from build123d import *

# Parameters (mm, degrees)
BOSS_EXTRUDE1_DEPTH = 15
SCALE1_SCALE        = 0.147347741
CUT_EXTRUDE1_REACH  = 182.668
SKETCH4_R           = 2.5


with BuildPart() as part:
    # Sketch3 → Boss-Extrude1 (new body)
    with BuildSketch(Plane(origin=(0, 0, 0), x_dir=(0, 0, -1), z_dir=(1, 0, 0))):
        with BuildLine():
            Line((0, -60), (0, -86.184781703))
            ThreePointArc((0, -86.184781703), (14.644660941, -121.540120762), (50, -136.184781703))
            Line((50, -136.184781703), (73.642909299, -136.184781703))
            ThreePointArc((73.642909299, -136.184781703), (108.573727492, -150.409958986), (123.628662427, -184.991264087))
            Line((123.628662427, -184.991264087), (125.683202704, -271.037537481))
            ThreePointArc((125.683202704, -271.037537481), (116.280768167, -291.592024429), (95.295179386, -299.98831959))
            Line((95.295179386, -299.98831959), (73.775693132, -299.98831959))
            ThreePointArc((73.775693132, -299.98831959), (63.169091414, -304.381717872), (58.775693132, -314.98831959))
            Line((58.775693132, -314.98831959), (58.775693132, -326.270417599))
            ThreePointArc((58.775693132, -326.270417599), (61.70462532, -333.341485411), (68.775693132, -336.270417599))
            Line((68.775693132, -336.270417599), (117.262564818, -336.270417599))
            Line((117.262564818, -336.270417599), (138.939006392, -336.270417599))
            ThreePointArc((138.939006392, -336.270417599), (153.081142016, -330.412553223), (158.939006392, -316.270417599))
            Line((158.939006392, -316.270417599), (158.939006392, -146.184781703))
            Line((158.939006392, -146.184781703), (158.939006392, -50))
            Line((158.939006392, -50), (158.939006392, -11.480346054))
            ThreePointArc((158.939006392, -11.480346054), (148.053108697, 21.328755123), (117.156078712, 36.830801017))
            ThreePointArc((117.156078712, 36.830801017), (39.60735059, 11.368133348), (0, -60))
        make_face()
    extrude(amount=BOSS_EXTRUDE1_DEPTH)


with BuildPart() as part_1:
    # Scale1: scaled about (7.5, -112.632543916, -97.960281801)
    add(part.part.scale(SCALE1_SCALE).moved(Location((6.394891943, -96.036393007, -83.52605557))))

    # Sketch4 → Cut-Extrude1 (cut, up to next)
    with BuildSketch(Plane(origin=(8.605108057, 0, 0), x_dir=(0, 0, -1), z_dir=(1, 0, 0)), mode=Mode.PRIVATE) as cut_extrude1_sk1:
        with Locations((96.192054569, -104.044147658)):
            Circle(SKETCH4_R)
    cut_extrude1_tool1 = extrude(cut_extrude1_sk1.sketch, amount=-CUT_EXTRUDE1_REACH, mode=Mode.PRIVATE) & part_1.part
    add(cut_extrude1_tool1.solids().sort_by_distance((8.605108, -104.044148, -96.192055))[0], mode=Mode.SUBTRACT)


solid = part_1.part
Here's how the part is built. I have some questions about the finished solid (model axes, mm). A direction names the side the tool comes from. Round coordinates to 2 decimals unless told otherwise and drop trailing zeros. Loops run counter-clockwise (first coordinate to the right, second up) from the corner with the lowest first, then second, coordinate; pieces in that order, holes last.
1. If we section it at B-B on x = 7.2: Write out the boundary of the cut face in (y, z), plus the area to 3 significant figures.
Answer list:
outline: (-145.59, -104) arc R2.95 ccw to (-142.64, -106.95) - (-97.73, -106.95) arc R6.65 ccw to (-90.61, -100.79) arc R16.48 ccw to (-104.88, -83.53) - (-108.74, -83.53) arc R7.37 ccw to (-116.1, -90.89) - (-116.1, -94.38) arc R7.37 cw to (-123.29, -101.74) - (-135.97, -102.05) arc R4.48 cw to (-140.24, -97.57) - (-140.24, -94.4) arc R2.21 ccw to (-142.45, -92.19) - (-144.11, -92.19) arc R1.47 ccw to (-145.59, -93.66) - close; hole circle Ø5 at (-104.04, -96.19)
area: 715 mm2
2. We'd pull the mould along Y, two halves only. Please class faces 1 (the face through (7, -120, -106.945)), 2 (the face through (7, -140.239, -96)), 3 (the face through (7.485, -144.745, -106.059)): +Y half, -Y half, draft (parallel to the pull), parting line (faces both ways), or undercut.
Answer list:
face 1: draft
face 2: undercut
face 3: -Y half
3. If we section it at C-C on y = -113: Write out the boundary of the cut face in (x, z).
Answer list:
outline: (6.39, -106.95) - (8.61, -106.95) - (8.61, -84.89) - (6.39, -84.89) - close
4. For P1, Ø1, axis at x = 8, y = -110.5, coming from the -Z side; P2, Ø0.5, axis at x = 8, y = -143, coming from the +Z side, each with a flat end and sliding along its axis, tell me the tip position at first contact or that it passes through.
Answer list:
P1: stops at z = -106.95
P2: stops at z = -92.19
5. If we section it at D-D on z = -104.5: Write out the boundary of the cut face in (x, y).
Answer list:
outline: (6.39, -145.54) - (8.61, -145.54) - (8.61, -92.08) - (6.39, -92.08) - close
6. If I drill on line 1 along Y through (x, z) = (6.6, -94.75); line 2 along Y through (x, z) = (6.85, -96.25); line 3 along Y through (x, z) = (8.45, -93.25), over which ranges is the centre line in solid material (lowest first)?
Answer list:
line 1: y = -145.59 to -140.24, -116.11 to -106.09, -102 to -91.4
line 2: y = -145.59 to -140.24, -116.34 to -106.54, -101.54 to -90.98
line 3: y = -145.53 to -140.56, -116.1 to -91.97
7. Which directions (+Z, -Z, +X, -X, +Y, -Y) give clear straight access to the entire face, cutting with the end or side of a thin tool? Please do faces 4 (the face through (7, -143, -92.187)), 5 (the face through (8.605, -112, -98)), 6 (the face through (7.485, -118.144, -99.467)).
Answer list:
face 4: +Z, +X, -X, -Y
face 5: +Z, -Z, +X, +Y, -Y
face 6: +Z, +X, -X
8. If we section it at A-A on z = -95.5: Write out the boundary of the cut face in (x, y).
Answer list:
outline: (6.39, -145.59) - (8.61, -145.59) - (8.61, -140.24) - (6.39, -140.24) - close; (6.39, -116.19) - (8.61, -116.19) - (8.61, -106.45) - (6.39, -106.45) - close; (6.39, -101.64) - (8.61, -101.64) - (8.61, -91.17) - (6.39, -91.17) - close
